Verification items for this drawing (mm, ordinates from the low corner). A direction names the side the tool comes from. Give positions to 0.01 mm unless a question says otherwise; leave off trailing zeros. Order: outer loops, then holes, each group sorted by start corner. A loop starts at its lowest first (then second) coordinate and runs counter-clockwise, first axis right, second up.
(1) Sectioned sample at C-C on z = 1.54. Record the cut outline in (x, y) (1 decimal).
(2) Gauge pin test, flat ends, axial feed: pin 1 (5 mm diameter, centred on y = 9, z = 4, fed in from +X); pin 2 (1.1 mm diameter, centred on x = 1, y = 15.5, fed in from -Z) (1 decimal); pin 3 (7.5 mm diameter, centred on x = 10.5, y = 9, fed in from -Z); pin 4 (8 mm diameter, centred on x = 13, z = 11, fed in from -Y). Record the tip position at first contact, or that the pin passes through.
(3) Access from +Z, -Z, +X, -X, +Y, -Y to the whole of each face (thin tool, end or side, straight path). Record for the marked faces 1, 2, 3, 4 and 5.
(4) Sectioned sample at A-A on z = 10.75. Record the cut outline in (x, y), plus the area to 3 significant figures.
(5) Sectioned sample at D-D on y = 22.75. Record the cut outline in (x, z) (1 decimal).
(6) Scan lines: L1, parallel to Z at x = 21.4, y = 12.7 (1 decimal); L2, parallel to X at y = 19.5, z = 11.5; L3, parallel to Z at x = 18.5, y = 18. Record each from-to range of solid material in increasing order.
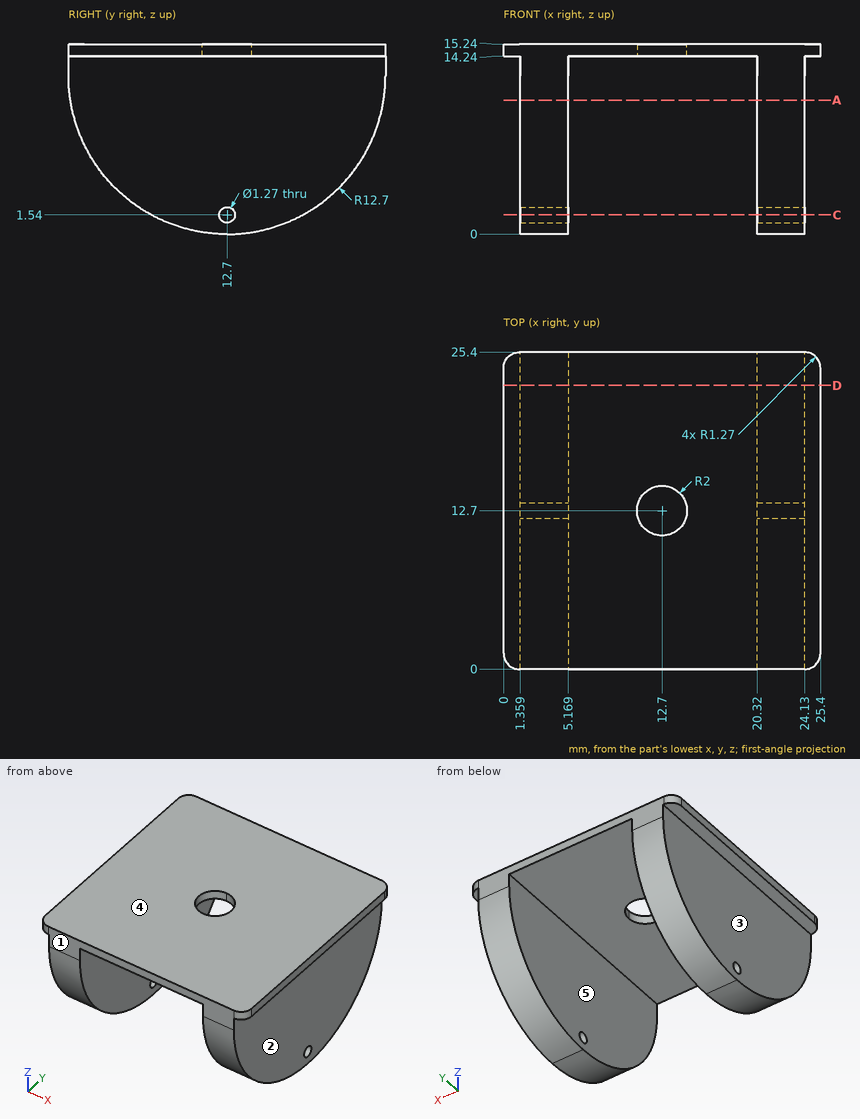
Ans:
1. outline: (1.4, 6.6) - (5.2, 6.6) - (5.2, 12.1) - (1.4, 12.1) - close; (1.4, 13.3) - (5.2, 13.3) - (5.2, 18.8) - (1.4, 18.8) - close; (20.3, 6.6) - (24.1, 6.6) - (24.1, 12.1) - (20.3, 12.1) - close; (20.3, 13.3) - (24.1, 13.3) - (24.1, 18.8) - (20.3, 18.8) - close
2. pin 1: stops at x = 24.13
2. pin 2: stops at z = 0.2
2. pin 3: stops at z = 14.24
2. pin 4: stops at y = 0
3. face 1: +Z, -Z, +X, -X, -Y
3. face 2: -Z, +X, +Y, -Y
3. face 3: -Z, -X, +Y, -Y
3. face 4: +Z, +X, -X, +Y, -Y
3. face 5: -Z, +Y, -Y
4. outline: (1.36, 0.15) - (5.17, 0.15) - (5.17, 25.25) - (1.36, 25.25) - close; (20.32, 0.15) - (24.13, 0.15) - (24.13, 25.25) - (20.32, 25.25) - close
4. area: 191 mm2
5. outline: (0, 14.2) - (1.4, 14.2) - (1.4, 4.9) - (5.2, 4.9) - (5.2, 14.2) - (20.3, 14.2) - (20.3, 4.9) - (24.1, 4.9) - (24.1, 14.2) - (25.4, 14.2) - (25.4, 15.2) - (0, 15.2) - close
6. L1: z = 0 to 0.9, 2.2 to 15.2
6. L2: x = 1.36 to 5.17, 20.32 to 24.13
6. L3: z = 14.24 to 15.24
